from build123d import *

# Parameters (mm, degrees)
F1_W     = 50
F1_H     = 50
F1_W_2   = 8.3333333333
F1_H_2   = 0.8333333333
F1_W_3   = 0.8333333333
F1_H_3   = 8.3333333333
F1_R     = 1.25
F2_DEPTH = 1
F3_R     = 5
F4_SIZE  = 5


with BuildPart() as f2:
    # F1 (on Top) → F2 (new body)
    with BuildSketch(Plane.XY):
        Rectangle(F1_W, F1_H)
        Polygon((-17.0833333333, -11.3915608176), (-10.8333333333, -15), (-17.0833333333, -18.6084391824), align=None, mode=Mode.SUBTRACT)
        Polygon((-5, -10.8333333333), (-0.8333333333, -15), (-5, -19.1666666667), (-9.1666666667, -15), align=None, mode=Mode.SUBTRACT)
        Polygon((-11.6290958568, -2.5508947821), (-10.8333333333, -5), (-11.6290958568, -7.4491052179), (-13.7124291901, -8.9627354846), (-16.2875708099, -8.9627354846), (-18.3709041432, -7.4491052179), (-19.1666666667, -5), (-18.3709041432, -2.5508947821), (-16.2875708099, -1.0372645154), (-13.7124291901, -1.0372645154), align=None, mode=Mode.SUBTRACT)
        Polygon((-1.8081481537, -2.321718293), (-0.8333333333, -5), (-1.8081481537, -7.678281707), (-4.2764659264, -9.1033656376), (-7.0833333333, -8.6084391824), (-8.9153859199, -6.4250839305), (-8.9153859199, -3.5749160695), (-7.0833333333, -1.3915608176), (-4.2764659264, -0.8966343624), align=None, mode=Mode.SUBTRACT)
        Polygon((6.2875708099, -11.0372645154), (9.1666666667, -15), (6.2875708099, -18.9627354846), (1.6290958568, -17.4491052179), (1.6290958568, -12.5508947821), align=None, mode=Mode.SUBTRACT)
        Polygon((17.0833333333, -11.3915608176), (19.1666666667, -15), (17.0833333333, -18.6084391824), (12.9166666667, -18.6084391824), (10.8333333333, -15), (12.9166666667, -11.3915608176), align=None, mode=Mode.SUBTRACT)
        Polygon((7.9462782549, -2.0537217451), (9.1666666667, -5), (7.9462782549, -7.9462782549), (5, -9.1666666667), (2.0537217451, -7.9462782549), (0.8333333333, -5), (2.0537217451, -2.0537217451), (5, -0.8333333333), align=None, mode=Mode.SUBTRACT)
        Polygon((17.5978741744, -1.742368823), (19.1666666667, -5), (17.5978741744, -8.257631177), (14.0728294418, -9.0621996341), (11.2459630504, -6.807848913), (11.2459630504, -3.192151087), (14.0728294418, -0.9378003659), align=None, mode=Mode.SUBTRACT)
        with BuildLine():
            ThreePointArc((-10.8333333333, 5), (-14.2952022322, 3.7792544571), (-17.0833333333, 1.3915608176))
            ThreePointArc((-17.0833333333, 1.3915608176), (-16.4095955357, 5), (-17.0833333333, 8.6084391824))
            ThreePointArc((-17.0833333333, 8.6084391824), (-14.2952022322, 6.2207455429), (-10.8333333333, 5))
        make_face(mode=Mode.SUBTRACT)
        with BuildLine():
            ThreePointArc((-5, 0.8333333333), (-6.4043221776, 3.5956778224), (-9.1666666667, 5))
            ThreePointArc((-9.1666666667, 5), (-6.4043221776, 6.4043221776), (-5, 9.1666666667))
            ThreePointArc((-5, 9.1666666667), (-3.5956778224, 6.4043221776), (-0.8333333333, 5))
            ThreePointArc((-0.8333333333, 5), (-3.5956778224, 3.5956778224), (-5, 0.8333333333))
        make_face(mode=Mode.SUBTRACT)
        with Locations((-5, 11.25)):
            Rectangle(F1_W_2, F1_H_2, mode=Mode.SUBTRACT)
        with Locations((-18.75, 15)):
            Rectangle(F1_W_3, F1_H_3, mode=Mode.SUBTRACT)
        with Locations((-17.5, 15)):
            Rectangle(F1_W_3, F1_H_3, mode=Mode.SUBTRACT)
        with Locations((-16.25, 15)):
            Rectangle(F1_W_3, F1_H_3, mode=Mode.SUBTRACT)
        with Locations((-15, 15)):
            Rectangle(F1_W_3, F1_H_3, mode=Mode.SUBTRACT)
        with Locations((-13.75, 15)):
            Rectangle(F1_W_3, F1_H_3, mode=Mode.SUBTRACT)
        with Locations((-12.5, 15)):
            Rectangle(F1_W_3, F1_H_3, mode=Mode.SUBTRACT)
        with Locations((-11.25, 15)):
            Rectangle(F1_W_3, F1_H_3, mode=Mode.SUBTRACT)
        with Locations((-5, 12.5)):
            Rectangle(F1_W_2, F1_H_2, mode=Mode.SUBTRACT)
        with Locations((-5, 13.75)):
            Rectangle(F1_W_2, F1_H_2, mode=Mode.SUBTRACT)
        with Locations((-5, 15)):
            Rectangle(F1_W_2, F1_H_2, mode=Mode.SUBTRACT)
        with Locations((-5, 16.25)):
            Rectangle(F1_W_2, F1_H_2, mode=Mode.SUBTRACT)
        with Locations((-5, 17.5)):
            Rectangle(F1_W_2, F1_H_2, mode=Mode.SUBTRACT)
        with Locations((-5, 18.75)):
            Rectangle(F1_W_2, F1_H_2, mode=Mode.SUBTRACT)
        with BuildLine():
            add(Edge.make_bspline(
                [(5, 9.1666666667), (3.5845240526, 9.1666666667), (2.8562676857, 7.1437323143)],
                knots=[0, 0, 0, 1.0303768265, 1.0303768265, 1.0303768265], degree=2, weights=[1, 0.8701999068, 1]))
            add(Edge.make_bspline(
                [(7.1437323143, 7.1437323143), (6.4154759474, 9.1666666667), (5, 9.1666666667)],
                knots=[5.2528084807, 5.2528084807, 5.2528084807, 6.2831853072, 6.2831853072, 6.2831853072], degree=2, weights=[1, 0.8701999068, 1]))
            add(Edge.make_bspline(
                [(9.1666666667, 5), (9.1666666667, 6.4154759474), (7.1437323143, 7.1437323143)],
                knots=[0, 0, 0, 1.0303768265, 1.0303768265, 1.0303768265], degree=2, weights=[1, 0.8701999068, 1]))
            add(Edge.make_bspline(
                [(7.1437323143, 2.8562676857), (9.1666666667, 3.5845240526), (9.1666666667, 5)],
                knots=[5.2528084807, 5.2528084807, 5.2528084807, 6.2831853072, 6.2831853072, 6.2831853072], degree=2, weights=[1, 0.8701999068, 1]))
            add(Edge.make_bspline(
                [(2.8562676857, 2.8562676857), (5, -3.0985442984), (7.1437323143, 2.8562676857)],
                knots=[2.1112158271, 2.1112158271, 2.1112158271, 4.1719694801, 4.1719694801, 4.1719694801], degree=2, weights=[1, 0.5144957554, 1]))
            add(Edge.make_bspline(
                [(2.8562676857, 7.1437323143), (-3.0985442984, 5), (2.8562676857, 2.8562676857)],
                knots=[2.1112158271, 2.1112158271, 2.1112158271, 4.1719694801, 4.1719694801, 4.1719694801], degree=2, weights=[1, 0.5144957554, 1]))
        make_face(mode=Mode.SUBTRACT)
        with BuildLine():
            ThreePointArc((12.3333333333, 4.1339745962), (11.8333333333, 5), (12.3333333333, 5.8660254038))
            Line((12.3333333333, 5.8660254038), (15.5833333333, 7.7424137787))
            ThreePointArc((15.5833333333, 7.7424137787), (16.5833333333, 7.7424137787), (17.0833333333, 6.8763883749))
            Line((17.0833333333, 6.8763883749), (17.0833333333, 3.1236116251))
            ThreePointArc((17.0833333333, 3.1236116251), (16.5833333333, 2.2575862213), (15.5833333333, 2.2575862213))
            Line((15.5833333333, 2.2575862213), (12.3333333333, 4.1339745962))
        make_face(mode=Mode.SUBTRACT)
        Polygon((3.75, 16.25), (3.75, 19.1666666667), (6.25, 19.1666666667), (6.25, 16.25), (9.1666666667, 16.25), (9.1666666667, 13.75), (6.25, 13.75), (6.25, 10.8333333333), (3.75, 10.8333333333), (3.75, 13.75), (0.8333333333, 13.75), (0.8333333333, 16.25), align=None, mode=Mode.SUBTRACT)
        with Locations((15, 12.5)):
            Circle(F1_R, mode=Mode.SUBTRACT)
        with Locations((12.5, 15)):
            Circle(F1_R, mode=Mode.SUBTRACT)
        with Locations((17.5, 15)):
            Circle(F1_R, mode=Mode.SUBTRACT)
        with Locations((15, 17.5)):
            Circle(F1_R, mode=Mode.SUBTRACT)
    extrude(amount=F2_DEPTH)

    # F3
    f3_edges = [f2.edges().sort_by_distance(p)[0] for p in [
        (-25, -25, 0.5),
        (25, 25, 0.5),
    ]]
    fillet(f3_edges, radius=F3_R)

    # F4
    f4_edges = [f2.edges().sort_by_distance(p)[0] for p in [
        (25, -25, 0.5),
        (-25, 25, 0.5),
    ]]
    chamfer(f4_edges, length=F4_SIZE)


solid = f2.part
Could you check a few things on this model? Use its own coordinates, in mm. Give positions to 0.01 mm unless a question says otherwise; leave off trailing zeros. Order: outer loops, then holes, each group sorted by start corner. A loop starts at its lowest first (then second) coordinate and runs counter-clockwise, first axis right, second up.
1. Suppose I cut it at C-C (x = 15). List the corners of the cut face in (y, z) for me.
2. Suppose I cut it at A-A (y = -13.5). List the corners of the cut face in (x, z) for me, plus the area to 3 significant figures.
3. I need wall thicknesses on L1, parallel to Y at x = 5.5, z = 0.5; L2, parallel to Y at x = 12, z = 0.35; L3, parallel to X at y = -4, z = 0.7. Which ranges of each line are inside material? Lowest first, please.
4. We'd pull the mould along X, two halves only. Please class faces 1 (the cylindrical face through (-23.57, -23.5, 0.51)), 2 (the flat face through (-17.34, -1.8, 0.49)): pulls with the +X half, pulls with the -X half, needs draft (parallel to the pull), parting line crosses it, or undercut.
5. Suppose I cut it at B-B (z = 0.45). Give the number of separate pieces and of enclosed holes in the cut face, plus the area to 3 significant figures.
Solved:
1. outline: (-25, 0) - (-18.61, 0) - (-18.61, 1) - (-25, 1) - close; (-11.39, 0) - (-8.85, 0) - (-8.85, 1) - (-11.39, 1) - close; (-1.15, 0) - (2.59, 0) - (2.59, 1) - (-1.15, 1) - close; (7.41, 0) - (11.25, 0) - (11.25, 1) - (7.41, 1) - close; (13.75, 0) - (16.25, 0) - (16.25, 1) - (13.75, 1) - close; (18.75, 0) - (25, 0) - (25, 1) - (18.75, 1) - close
2. outline: (-25, 0) - (-17.08, 0) - (-17.08, 1) - (-25, 1) - close; (-13.43, 0) - (-7.67, 0) - (-7.67, 1) - (-13.43, 1) - close; (-2.33, 0) - (1.63, 0) - (1.63, 1) - (-2.33, 1) - close; (8.08, 0) - (11.7, 0) - (11.7, 1) - (8.08, 1) - close; (18.3, 0) - (25, 0) - (25, 1) - (18.3, 1) - close
2. area: 28.0 mm2
3. L1: y = -25 to -18.71, -11.29 to -8.96, -1.04 to 0.92, 9.08 to 10.83, 19.17 to 25
3. L2: y = -25 to -17.02, -12.98 to -7.41, -2.59 to 4.45, 5.55 to 13.85, 16.15 to 25
3. L3: x = -25 to -18.84, -11.16 to -8.92, -1.2 to 1.25, 8.75 to 11.25, 18.69 to 25
4. face 1: pulls with the -X half
4. face 2: undercut
5. separate pieces: 1
5. enclosed holes: 31
5. area: 1,870 mm2
